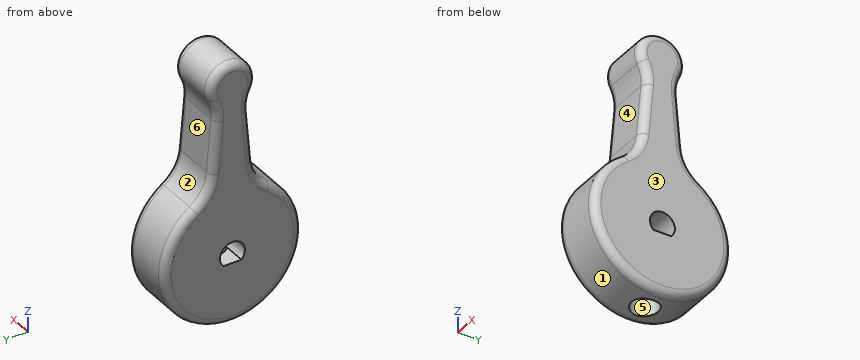
```python
from build123d import *

# Parameters (mm, degrees)
BOSS_EXTRUDE1_DEPTH = 3.5
FILLET1_R           = 5
HOLE1_D             = 2.5
HOLE1_DEPTH         = 9
HOLE1_CBORE_D       = 3.5
HOLE1_CBORE_DEPTH   = 3
FILLET2_R           = 1


with BuildPart() as part:
    # Sketch1 → Boss-Extrude1 (new, symmetric)
    with BuildSketch(Plane(origin=(0, 0, 0), x_dir=(0, 0, -1), z_dir=(1, 0, 0))):
        with BuildLine():
            Line((-19.763932023, 2), (-8.485281374, 3))
            ThreePointArc((-8.485281374, 3), (9, 0), (-8.485281374, -3))
            Line((-8.485281374, -3), (-19.763932023, -2))
            ThreePointArc((-19.763932023, -2), (-25, 0), (-19.763932023, 2))
        make_face()
        with BuildLine():
            Line((1.125, -1.17260394), (1.125, 1.17260394))
            ThreePointArc((1.125, 1.17260394), (-1.625, 0), (1.125, -1.17260394))
        make_face(mode=Mode.SUBTRACT)
    extrude(amount=BOSS_EXTRUDE1_DEPTH, both=True)

    # Fillet1
    fillet1_edges = [part.edges().sort_by_distance(p)[0] for p in [
        (0, 2, 19.763932023),
        (0, 3, 8.485281374),
        (0, -3, 8.485281374),
        (0, -2, 19.763932023),
    ]]
    fillet(fillet1_edges, radius=FILLET1_R)

    # Hole1
    with Locations(Plane(origin=(0, 0, -9.125), x_dir=(1, 0, 0), z_dir=(0, 0, -1))):
        with Locations((0, 0)):
            CounterBoreHole(HOLE1_D / 2, HOLE1_CBORE_D / 2, HOLE1_CBORE_DEPTH, depth=HOLE1_DEPTH)

    # Fillet2
    fillet2_edges = [part.edges().sort_by_distance(p)[0] for p in [
        (-3.5, 0, 25),
        (3.5, 0, 25),
        (-3.5, 2.458817952, 14.589084631),
        (3.5, 2.458817952, 14.589084631),
        (-3.5, 0, -9),
        (3.5, 0, -9),
        (-3.5, -2.458817952, 14.589084631),
        (3.5, -2.458817952, 14.589084631),
        (-3.5, 2.230698388, 19.336127101),
        (3.5, 2.230698388, 19.336127101),
        (-3.5, -3.440789323, 9.110481838),
        (3.5, -3.440789323, 9.110481838),
        (-3.5, -2.230698388, 19.336127101),
        (3.5, -2.230698388, 19.336127101),
        (-3.5, 3.440789323, 9.110481838),
        (3.5, 3.440789323, 9.110481838),
    ]]
    fillet(fillet2_edges, radius=FILLET2_R)


solid = part.part
```
Work out the finished part from the listing and answer in its coordinate system (mm). Face numbers are marked on the shaded views. A direction names the side the tool comes from. Round coordinates to 2 decimals unless told otherwise and drop trailing zeros. Loops run counter-clockwise (first coordinate to the right, second up) from the corner with the lowest first, then second, coordinate; pieces in that order, holes last. Notation, with made-up numbers: M -11,16 L 36,16 A38 cw 36,55 Z; hole C 59.5,15 d6. An arc over 180 degrees is marked long. Use CSV: the item, a comma, the result in double quotes.
Q1. A tool of negligible diameter and unlimited length cuts with its end or side. For the marked faces 4, 5 and 6, from which of +Z, -Z, +X, -X, +Y, -Y can it reach the whole face along a straight path? Write none if from no direction.
Determined:
face 4,"+X, -X, -Y"
face 5,"-Z"
face 6,"+X, -X, +Y"
Q2. Consider L1, parallel to Z at x = 3, y = -6; L2, parallel to Y at x = 0.75, z = -1; L3, parallel to Y at x = 0, z = -3.85. Determine where each line is inside the solid, lowest interval first.
Determined:
L1,"-6.53 to 6.53"
L2,"-8.94 to -1.28, 1.28 to 8.94"
L3,"-8.13 to -1.25, 1.25 to 8.13"
Q3. The mould has two halves that part along Z. Classify the marked faces 1, 2 and 3: pulls with the +Z half, pulls with the -Z half, needs draft (parallel to the pull), parting line crosses it, or undercut.
Determined:
face 1,"parting line crosses it"
face 2,"undercut"
face 3,"needs draft"
Q4. Section A-A, the plane y = 0 is taken. Determine the outline of the cut face in (x, z) (3 decimals).
Determined:
outline,"M -3.5,-8 A1 ccw -2.5,-9 L -1.75,-9 L -1.75,-6.125 L -1.25,-6.125 L -1.25,-1.125 L -3.5,-1.125 Z; M -3.5,1.625 L 3.5,1.625 L 3.5,24 A1 ccw 2.5,25 L -2.5,25 A1 ccw -3.5,24 Z; M 1.25,-6.125 L 1.75,-6.125 L 1.75,-9 L 2.5,-9 A1 ccw 3.5,-8 L 3.5,-1.125 L 1.25,-1.125 Z"
Q5. Section B-B, the plane x = 0 is taken. Determine the outline of the cut face in (y, z) (3 decimals), then the cut area to 3 significant figures.
Determined:
outline,"M -4.974,7.501 A9 ccw -1.75,-8.828 L -1.75,-6.125 L -1.25,-6.125 L -1.25,-1.038 A1.625 cw long 1.25,-1.038 L 1.25,-6.125 L 1.75,-6.125 L 1.75,-8.828 A9 ccw 4.974,7.501 A5 cw 2.757,11.226 L 2.161,17.952 A5 cw 2.678,20.648 A3 ccw long -2.678,20.648 A5 cw -2.161,17.952 L -2.757,11.226 A5 cw Z"
area,"308 mm2"
Q6. Each of these flat-tipped pins is pushed along its axis until it touches: pin 1 (3 mm diameter, centred on x = -0.5, z = 1.5, fed in from +Y); pin 2 (1 mm diameter, centred on x = 1, y = 0, fed in from -Z) (3 decimals); pin 3 (3 mm diameter, centred on x = -1.5, y = 3.5, fed in from +Z); pin 4 (2 mm diameter, centred on x = 0, y = 0, fed in from -Z). Where does it stop, or does it pass through?
Determined:
pin 1,"y = 9"
pin 2,"z = -6.125"
pin 3,"z = 24.24"
pin 4,"z = 1.28"
